The drawing under review shows one solid part. Ordinate dimensions are in mm from its lowest x, y, z. A direction names the side the tool comes from. Coordinates: 2 decimals unless noted, no trailing zeros. Order: outer loops, then holes, each group sorted by start corner. A loop starts at its lowest first (then second) coordinate and runs counter-clockwise, first axis right, second up.
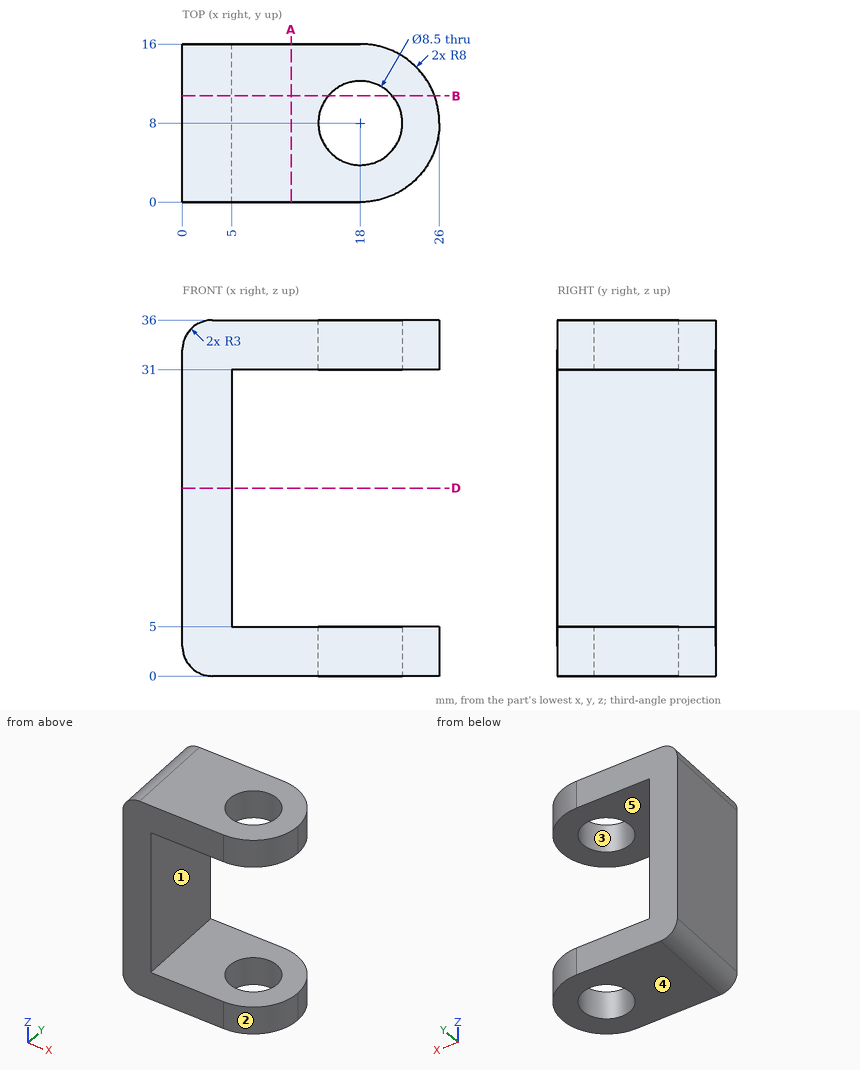
1. Add section D-D (z = 19). Give the boundary of the cut face in (x, y).
2. Add section A-A (x = 11). Give the boundary of the cut face in (y, z).
3. For the marked faces 4 and 5, list the 3-axis set-ups (+Z, -Z, +X, -X, +Y, -Y) from which the entire face can be reached by the end or side of a thin tool; tool diameter is ignored.
4. Add section B-B (y = 10.75). Give the boundary of the cut face in (x, z), and give its area (3 significant figures).
5. Mouldability with a two-part tool opening along Y and no side actions: class the marked faces 1, 2 and 3 as pulls with the +Y half, pulls with the -Y half, needs draft (parallel to the pull), parting line crosses it, or undercut.
6. To check wall thickness, follow line 1 (Z direction, x = 19.75, y = 12); line 2 (Y direction, x = 18, z = 2.1); line 3 (X direction, y = 7.75, z = 4.5). State the ranges of each line that lie inside material, in increasing order.
7. Insertion check: pin 1 (5 mm diameter, centred on x = 18, y = 8, fed in from +Z); pin 2 (1.5 mm diameter, centred on y = 11.5, z = 18, fed in from +X). Each pin has a flat end and moves straight along its axis. Give the tip position at first contact, or say it passes through.
Solution:
1. outline: (0, 0) - (5, 0) - (5, 16) - (0, 16) - close
2. outline: (0, 0) - (16, 0) - (16, 5) - (0, 5) - close; (0, 31) - (16, 31) - (16, 36) - (0, 36) - close
3. face 4: -Z, +X, -X, +Y, -Y
3. face 5: +X, +Y, -Y
4. outline: (0, 3) arc R3 ccw to (3, 0) - (14.76, 0) - (14.76, 5) - (5, 5) - (5, 31) - (14.76, 31) - (14.76, 36) - (3, 36) arc R3 ccw to (0, 33) - close; (21.24, 0) - (25.51, 0) - (25.51, 5) - (21.24, 5) - close; (21.24, 31) - (25.51, 31) - (25.51, 36) - (21.24, 36) - close
4. area: 316 mm2
5. face 1: needs draft
5. face 2: pulls with the -Y half
5. face 3: undercut
6. line 1: z = 0 to 5, 31 to 36
6. line 2: y = 0 to 3.75, 12.25 to 16
6. line 3: x = 0 to 13.76, 22.24 to 26
7. pin 1: passes through
7. pin 2: stops at x = 5
